from build123d import *

# Parameters (mm, degrees)
BOX_W           = 33
BOX_H           = 33
BOX_DEPTH       = 50
SKETCH002_R     = 9
PAD001_DEPTH    = 2.5
SKETCH003_R     = 3.5
POCKET001_DEPTH = 53


with BuildPart() as part:
    # Box → Box (new body)
    with BuildSketch(Plane(origin=(-16.5, -16.5, 25), x_dir=(1, 0, 0), z_dir=(0, 0, 1))):
        with Locations((16.5, 16.5)):
            Rectangle(BOX_W, BOX_H)
    extrude(amount=BOX_DEPTH)

    # Sketch002 → Pad001 (new body)
    with BuildSketch(Plane(origin=(-16.5, -16.5, 25), x_dir=(1, 0, 0), z_dir=(0, 0, -1))):
        with Locations((16.5, -16.5)):
            Circle(SKETCH002_R)
    extrude(amount=PAD001_DEPTH)

    # Sketch003 → Pocket001 (cut)
    with BuildSketch(Plane(origin=(-16.5, -16.5, 22.5), x_dir=(1, 0, 0), z_dir=(0, 0, -1))):
        with Locations((16.5, -16.5)):
            Circle(SKETCH003_R)
    extrude(amount=-POCKET001_DEPTH, mode=Mode.SUBTRACT)


solid = part.part
Design review of the part built by this model. Coordinates are the model's own, in mm. A direction names the side the tool comes from. Round coordinates to 2 decimals unless told otherwise and drop trailing zeros. Loops run counter-clockwise (first coordinate to the right, second up) from the corner with the lowest first, then second, coordinate; pieces in that order, holes last. Notation, with made-up numbers: (82, 53.5) -> (104, 53.5) arc R27 cw to (104, 70.5) -> close; hole circle Ø4 at (81, 58.5). An arc over 180 degrees is marked (long way). Use one line per item in the form item = value. Start each with the question number.
Q1. Wall thickness on line 1 along Y through (x, z) = (0, 61); line 2 along Z through (x, y) = (3, 13.5): over which ranges is each line inside the solid? List them lowest first. Write a range as [from, to].
Q2. For pin 1 Ø3 at (x, y) = (12.5, -13) entering from -Z; pin 2 Ø8 at (x, y) = (0, 0) entering from -Z, all flat-tipped, find the tip position at first contact; note any pin that passes through.
Q3. Machinability: for faces 1 (the face through (0, -16.5, 50)), 2 (the face through (7, 8, 25)), which of the approach directions +Z, -Z, +X, -X, +Y, -Y give a long, thin tool a straight path to every point of the face, cutting with its end or side? Answer none if there is none.
Q4. We need section C-C on z = 69. Give the boundary of the cut face in (x, y).
Q5. We need section D-D on y = -7. Give the boundary of the cut face in (x, z), then the cut area to 3 significant figures.
Q6. We need section A-A on y = 0. Give the boundary of the cut face in (x, z), then the cut area to 3 significant figures.
Q7. Draft analysis for pull direction X (two halves, no side actions). For faces 3 (the face through (0, 4, 22.5)), 4 (the face through (3.233, 1.341, 48.382)), 5 (the face through (16.5, 0, 50)), state which applies: +X half, -X half, draft (parallel to the pull), parting line (faces both ways), or undercut.
Calculated:
q1.line_1 = [-16.5, -3.5], [3.5, 16.5]
q1.line_2 = [25, 75]
q2.pin_1 = 25
q2.pin_2 = 22.5
q3.face_1 = +Z, -Z, +X, -X, -Y
q3.face_2 = -Z
q4.outline = (-16.5, -16.5) -> (16.5, -16.5) -> (16.5, 16.5) -> (-16.5, 16.5) -> close; hole circle Ø7 at (0, 0)
q5.outline = (-16.5, 25) -> (-5.66, 25) -> (-5.66, 22.5) -> (5.66, 22.5) -> (5.66, 25) -> (16.5, 25) -> (16.5, 75) -> (-16.5, 75) -> close
q5.area = 1,680 mm²
q6.outline = (-16.5, 25) -> (-9, 25) -> (-9, 22.5) -> (-3.5, 22.5) -> (-3.5, 75) -> (-16.5, 75) -> close; (3.5, 22.5) -> (9, 22.5) -> (9, 25) -> (16.5, 25) -> (16.5, 75) -> (3.5, 75) -> close
q6.area = 1,330 mm²
q7.face_3 = draft
q7.face_4 = undercut
q7.face_5 = +X half
